from build123d import *

# Parameters (mm, degrees)
BOSS_EXTRUDE1_DEPTH = 10
SKETCH2_W           = 3
SKETCH2_H           = 122
BOSS_EXTRUDE2_DEPTH = 1.25
SKETCH3_W           = 6
SKETCH3_H           = 10
BOSS_EXTRUDE3_DEPTH = 3
SKETCH4_W           = 122
SKETCH4_H           = 5.15
BOSS_EXTRUDE4_DEPTH = 52
CUT_EXTRUDE1_DEPTH  = 52
BOSS_EXTRUDE6_START = 20
BOSS_EXTRUDE6_DEPTH = 20


with BuildPart() as part:
    # Sketch1 → Boss-Extrude1 (new body)
    with BuildSketch(Plane(origin=(0, 0, 0), x_dir=(1, 0, 0), z_dir=(0, 1, 0))):
        Polygon((-28.5, 64), (28.5, 64), (28.5, -61), (25.5, -61), (25.5, 61), (-25.5, 61), (-25.5, -61), (-28.5, -61), align=None)
    extrude(amount=BOSS_EXTRUDE1_DEPTH)

    # Sketch2 → Boss-Extrude2 (add)
    with BuildSketch(Plane.XZ):
        with Locations((-24, 0)):
            Rectangle(SKETCH2_W, SKETCH2_H)
        with Locations((24, 0)):
            Rectangle(SKETCH2_W, SKETCH2_H)
    extrude(amount=-BOSS_EXTRUDE2_DEPTH)

    # Sketch3 → Boss-Extrude3 (add)
    with BuildSketch(Plane.XY.offset(61)):
        with Locations((-25.5, 5)):
            Rectangle(SKETCH3_W, SKETCH3_H)
        with Locations((25.5, 5)):
            Rectangle(SKETCH3_W, SKETCH3_H)
    extrude(amount=BOSS_EXTRUDE3_DEPTH)

    # Sketch4 → Boss-Extrude4 (add)
    with BuildSketch(Plane(origin=(-25.5, 0, 0), x_dir=(0, 0, -1), z_dir=(1, 0, 0))):
        with Locations((0, 7.425)):
            Rectangle(SKETCH4_W, SKETCH4_H)
    extrude(amount=BOSS_EXTRUDE4_DEPTH)

    # Sketch5 → Cut-Extrude1 (cut)
    with BuildSketch(Plane(origin=(0, 10, 0), x_dir=(1, 0, 0), z_dir=(0, 1, 0))):
        with BuildLine():
            Line((-22, 15.667860965), (-22, -15.667860965))
            ThreePointArc((-22, -15.667860965), (-21.711009048, -16.952551567), (-20.899713371, -17.989732863))
            Line((-20.899713371, -17.989732863), (-1.899713371, -33.535187408))
            ThreePointArc((-1.899713371, -33.535187408), (0, -34.213315511), (1.899713371, -33.535187408))
            Line((1.899713371, -33.535187408), (20.899713371, -17.989732863))
            ThreePointArc((20.899713371, -17.989732863), (21.711009048, -16.952551567), (22, -15.667860965))
            Line((22, -15.667860965), (22, 15.667860965))
            ThreePointArc((22, 15.667860965), (21.771638598, 16.815911262), (21.121320344, 17.789181309))
            Line((21.121320344, 17.789181309), (14.878679656, 24.031821996))
            ThreePointArc((14.878679656, 24.031821996), (13.90540961, 24.68214025), (12.757359313, 24.910501652))
            Line((12.757359313, 24.910501652), (-12.757359313, 24.910501652))
            ThreePointArc((-12.757359313, 24.910501652), (-13.90540961, 24.68214025), (-14.878679656, 24.031821996))
            Line((-14.878679656, 24.031821996), (-21.121320344, 17.789181309))
            ThreePointArc((-21.121320344, 17.789181309), (-21.771638598, 16.815911262), (-22, 15.667860965))
        make_face()
    extrude(amount=-CUT_EXTRUDE1_DEPTH, mode=Mode.SUBTRACT)

    # Sketch6 → Boss-Extrude6 (add)
    with BuildSketch(Plane(origin=(0, 10, 0), x_dir=(1, 0, 0), z_dir=(0, 1, 0)).offset(BOSS_EXTRUDE6_START)):
        with BuildLine():
            Line((-22.166188951, -19.537647461), (-3.166188951, -35.083102007))
            ThreePointArc((-3.166188951, -35.083102007), (0, -36.213315511), (3.166188951, -35.083102007))
            Line((3.166188951, -35.083102007), (22.166188951, -19.537647461))
            ThreePointArc((22.166188951, -19.537647461), (23.518348413, -17.809011969), (24, -15.667860965))
            Line((24, -15.667860965), (24, 15.667860965))
            ThreePointArc((24, 15.667860965), (23.619397663, 17.581278127), (22.535533906, 19.203394871))
            Line((22.535533906, 19.203394871), (16.292893219, 25.446035558))
            ThreePointArc((16.292893219, 25.446035558), (14.670776475, 26.529899315), (12.757359313, 26.910501652))
            Line((12.757359313, 26.910501652), (-12.757359313, 26.910501652))
            ThreePointArc((-12.757359313, 26.910501652), (-14.670776475, 26.529899315), (-16.292893219, 25.446035558))
            Line((-16.292893219, 25.446035558), (-22.535533906, 19.203394871))
            ThreePointArc((-22.535533906, 19.203394871), (-23.619397663, 17.581278127), (-24, 15.667860965))
            Line((-24, 15.667860965), (-24, -15.667860965))
            ThreePointArc((-24, -15.667860965), (-23.518348413, -17.809011969), (-22.166188951, -19.537647461))
        make_face()
        with BuildLine():
            Line((-20.899713371, -17.989732863), (-1.899713371, -33.535187408))
            ThreePointArc((-1.899713371, -33.535187408), (0, -34.213315511), (1.899713371, -33.535187408))
            Line((1.899713371, -33.535187408), (20.899713371, -17.989732863))
            ThreePointArc((20.899713371, -17.989732863), (21.711009048, -16.952551567), (22, -15.667860965))
            Line((22, -15.667860965), (22, 15.667860965))
            ThreePointArc((22, 15.667860965), (21.771638598, 16.815911262), (21.121320344, 17.789181309))
            Line((21.121320344, 17.789181309), (14.878679656, 24.031821996))
            ThreePointArc((14.878679656, 24.031821996), (13.90540961, 24.68214025), (12.757359313, 24.910501652))
            Line((12.757359313, 24.910501652), (-12.757359313, 24.910501652))
            ThreePointArc((-12.757359313, 24.910501652), (-13.90540961, 24.68214025), (-14.878679656, 24.031821996))
            Line((-14.878679656, 24.031821996), (-21.121320344, 17.789181309))
            ThreePointArc((-21.121320344, 17.789181309), (-21.771638598, 16.815911262), (-22, 15.667860965))
            Line((-22, 15.667860965), (-22, -15.667860965))
            ThreePointArc((-22, -15.667860965), (-21.711009048, -16.952551567), (-20.899713371, -17.989732863))
        make_face(mode=Mode.SUBTRACT)
    extrude(amount=-BOSS_EXTRUDE6_DEPTH)


solid = part.part
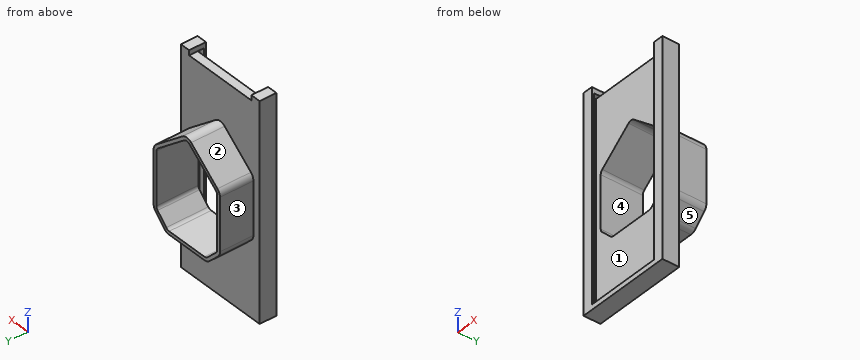
CAD build for the part. Positions are in the model's coordinates, mm. Face numbers are marked on the shaded views. A direction names the side the tool comes from. Round coordinates to 2 decimals unless told otherwise and drop trailing zeros. Loops run counter-clockwise (first coordinate to the right, second up) from the corner with the lowest first, then second, coordinate; pieces in that order, holes last. Notation, with made-up numbers: M 84,49.25 L 99,49.25 A17 cw 99,54.25 Z; hole C -32.5,5.25 d2. An arc over 180 degrees is marked long. One line per question, with ' | ' between items. Start each with the question number.
Item 1: Pin check, flat tips, straight feed: pin 1 Ø3.5 at (x, z) = (24.5, 11.5) entering from +Y; pin 2 Ø10 at (x, y) = (-21.5, 26.5) entering from +Z; pin 3 Ø6 at (y, z) = (18.5, 2.5) entering from +X; pin 4 Ø4 at (x, y) = (-7.5, 1.5) entering from +Z. Stop position of each tip, or through.
Item 2: Which spindle directions (+Z, -Z, +X, -X, +Y, -Y) get a long thin tool onto all of the face, cutting with end or side? Do the marked faces 1, 2, 3, 4 and 5. Say none if no direction does.
Item 3: Cut at C-C, the plane z = -48.5. Write the cut outline in (x, y), plus the area to 3 significant figures.
Item 4: Wall check: line 1 (X direction, y = 7, z = 0); line 2 (X direction, y = 4.75, z = -1); line 3 (Y direction, x = -23, z = -31.5). Give the ranges that are in metal, low to high.
Item 5: Cut at D-D, the plane z = 29. Write the cut outline in (x, y), plus the area to 3 significant figures.
Item 6: Cut at B-B, the plane y = 18.5. Write the cut outline in (x, z), plus the area to 3 significant figures.
Item 7: Cut at A-A, the plane x = 0. Write the cut outline in (y, z), plus the area to 3 significant figures.
Responses:
1) pin 1: stops at y = 30 | pin 2: stops at z = 24.17 | pin 3: stops at x = 24 | pin 4: stops at z = -61
2) face 1: none | face 2: +Z, -X, +Y | face 3: +Z, -Z, -X, +Y | face 4: +Y, -Y | face 5: -Z, +X, +Y
3) outline: M -28.5,0 L -22.5,0 L -22.5,1.25 L -25.5,1.25 L -25.5,4.85 L 25.5,4.85 L 25.5,1.25 L 22.5,1.25 L 22.5,0 L 28.5,0 L 28.5,10 L -28.5,10 Z | area: 330 mm²
4) line 1: x = -28.5 to -22, 22 to 28.5 | line 2: x = -28.5 to -25.5, 25.5 to 28.5 | line 3: y = 0 to 1.25, 4.85 to 10
5) outline: M -28.5,0 L -22.5,0 L -22.5,1.25 L -25.5,1.25 L -25.5,4.85 L -7.44,4.85 L -7.44,30 L -10.6,30 L -10.6,10 L -28.5,10 Z; M 7.44,4.85 L 25.5,4.85 L 25.5,1.25 L 22.5,1.25 L 22.5,0 L 28.5,0 L 28.5,10 L 10.6,10 L 10.6,30 L 7.44,30 Z | area: 380 mm²
6) outline: M -24,-15.67 A5 ccw -22.54,-19.2 L -16.29,-25.45 A5 ccw -12.76,-26.91 L 12.76,-26.91 A5 ccw 16.29,-25.45 L 22.54,-19.2 A5 ccw 24,-15.67 L 24,15.67 A5 ccw 22.17,19.54 L 3.17,35.08 A5 ccw -3.17,35.08 L -22.17,19.54 A5 ccw -24,15.67 Z; hole M -22,-15.67 A3 ccw -21.12,-17.79 L -14.88,-24.03 A3 ccw -12.76,-24.91 L 12.76,-24.91 A3 ccw 14.88,-24.03 L 21.12,-17.79 A3 ccw 22,-15.67 L 22,15.67 A3 ccw 20.9,17.99 L 1.9,33.54 A3 ccw -1.9,33.54 L -20.9,17.99 A3 ccw -22,15.67 Z | area: 360 mm²
7) outline: M 0,-64 L 10,-64 L 10,-26.91 L 30,-26.91 L 30,-24.91 L 4.85,-24.91 L 4.85,-61 L 0,-61 Z; M 4.85,34.21 L 30,34.21 L 30,36.21 L 10,36.21 L 10,61 L 4.85,61 Z | area: 434 mm²
